```python
from build123d import *

# Parameters (mm, degrees)
F0_W     = 100
F0_H     = 50
F0_H_2   = 30
F1_DEPTH = 80
F2_W     = 95
F2_H     = 38.437796
F2_H_2   = 26.119551
F3_DEPTH = 77
F5_DEPTH = 250


with BuildPart() as f1:
    # F0 (on Top) → F1 (new body)
    with BuildSketch(Plane.XY):
        with Locations((-4.275286, 7.339517)):
            Rectangle(F0_W, F0_H)
        with Locations((-4.275286, -32.660483)):
            Rectangle(F0_W, F0_H_2)
    extrude(amount=F1_DEPTH)

    # F2 (on face) → F3 (cut)
    with BuildSketch(Plane.XY.offset(80)):
        with Locations((-4.275286, 10.620619)):
            Rectangle(F2_W, F2_H)
        with Locations((-4.275286, -32.100707)):
            Rectangle(F2_W, F2_H_2)
    extrude(amount=-F3_DEPTH, mode=Mode.SUBTRACT)

    # F4 (on face) → F5 (cut)
    with BuildSketch(Plane(origin=(-54.275286, 0, 0), x_dir=(0, -1, 0), z_dir=(-1, 0, 0))):
        Polygon((-32.339517, 33.811978), (47.660483, 80), (-32.339517, 80), align=None)
    extrude(amount=-F5_DEPTH, mode=Mode.SUBTRACT)


solid = f1.part
```
Verification items for the finished model (mm, model axes). A direction names the side the tool comes from. Round coordinates to 2 decimals unless told otherwise and drop trailing zeros. Write each loop counter-clockwise with the first axis right and the second up, starting at its lowest first coordinate (ties: lowest second). Pieces come first, ordered by that corner, then holes. Notation, with made-up numbers: (8, 85) - (36, 85) arc R28 cw to (36, 121) - close; hole circle Ø3 at (82, 18). An arc over 180 degrees is marked (long way). Answer as a JSON object with one key per item and string values. Group by question number.
Q1. Section check D-D, the plane y = -1.5. Enter the section's corners in (x, z).
Q2. Section check B-B, the plane x = 15. Enter the section's corners in (y, z), plus the area to 3 significant figures.
Q3. Section check A-A, the plane z = 27. Enter the section's corners in (x, y), plus the area to 3 significant figures.
Q4. Tool access check on faces 5 (the flat face through (-5, -47.66, 39)), 6 (the flat face through (-5, 11, 3)). Record the directions out of +Z, -Z, +X, -X, +Y, -Y that give a thin tool (end or side, any length) a straight path to the whole face; none if there is none.
Q5. Go/stop test with flat-tipped pins: pin 1 Ø4 at (x, y) = (-39.5, 2.5) entering from +Z; pin 2 Ø12 at (y, z) = (14.5, 53) entering from -X; pin 3 Ø6 at (x, z) = (-4.5, 57.5) entering from +Y. Record where each tip stops, or that it passes through.
Q6. Mould release check, pull along X, two halves, no side actions. Record for faces 1 (the flat face through (-5, -7, 0)), 2 (the flat face through (-54.275, -16, 31)), 3 (the flat face through (45.725, -17, 31)), 4 (the flat face through (-5, -32, 3)): released by +X, released by -X, zero draft, split by the parting line, or undercut.
Q7. Section check C-C, the plane z = 60.5. Enter the section's corners in (x, y), plus the area to 3 significant figures.
Q8. Thickness scan on line 1 (Y direction, x = 15, z = 21.5); line 2 (X direction, y = 5, z = 6); line 3 (Y direction, x = 33.5, z = 44). Record the ranges inside material, lowest first.
Found:
{
 "1": {"outline": "(-54.28, 0) - (45.72, 0) - (45.72, 53.35) - (43.22, 53.35) - (43.22, 3) - (-51.78, 3) - (-51.78, 53.35) - (-54.28, 53.35) - close"},
 "2": {"outline": "(-47.66, 0) - (32.34, 0) - (32.34, 33.81) - (29.84, 35.26) - (29.84, 3) - (-8.6, 3) - (-8.6, 57.45) - (-19.04, 63.48) - (-19.04, 3) - (-45.16, 3) - (-45.16, 78.56) - (-47.66, 80) - close", "area": "1,110 mm^2"},
 "3": {"outline": "(-54.28, -47.66) - (45.72, -47.66) - (45.72, 32.34) - (-54.28, 32.34) - close; hole (-51.78, -45.16) - (43.22, -45.16) - (43.22, -19.04) - (-51.78, -19.04) - close; hole (-51.78, -8.6) - (43.22, -8.6) - (43.22, 29.84) - (-51.78, 29.84) - close", "area": "1,870 mm^2"},
 "4": {"face 5": "+Z, -Z, +X, -X, -Y", "face 6": "+Z"},
 "5": {"pin 1": "stops at z = 3", "pin 2": "passes through", "pin 3": "stops at y = -8.6"},
 "6": {"face 1": "zero draft", "face 2": "released by -X", "face 3": "released by +X", "face 4": "undercut"},
 "7": {"outline": "(-54.28, -47.66) - (45.72, -47.66) - (45.72, -13.89) - (-54.28, -13.89) - close; hole (-51.78, -45.16) - (43.22, -45.16) - (43.22, -19.04) - (-51.78, -19.04) - close", "area": "896 mm^2"},
 "8": {"line 1": "y = -47.66 to -45.16, -19.04 to -8.6, 29.84 to 32.34", "line 2": "x = -54.28 to -51.78, 43.22 to 45.72", "line 3": "y = -47.66 to -45.16, -19.04 to -8.6"}
}
